```python
from build123d import *

# Parameters (mm, degrees)
SKETCH1_W           = 35.5
SKETCH1_H           = 35
SKETCH1_W_2         = 23.5
SKETCH1_H_2         = 20.5
BOSS_EXTRUDE1_DEPTH = 10
SKETCH1_2_W         = 23.5
SKETCH1_2_H         = 20.5
BOSS_EXTRUDE2_DEPTH = 3.5
SKETCH2_R           = 2.75
SKETCH2_R_2         = 1.5
CUT_EXTRUDE1_DEPTH  = 5.5
SKETCH2_2_R         = 1.5
CUT_EXTRUDE2_DEPTH  = 41.822787754
CUT_EXTRUDE3_START  = -30
SKETCH2_3_R         = 2.75
SKETCH2_3_R_2       = 1.5
CUT_EXTRUDE3_DEPTH  = 5.5
BOSS_EXTRUDE3_DEPTH = 5


with BuildPart() as part:
    # Sketch1 → Boss-Extrude1 (new body)
    with BuildSketch(Plane(origin=(0, 0, 0), x_dir=(1, 0, 0), z_dir=(0, 1, 0))):
        Rectangle(SKETCH1_W, SKETCH1_H)
        Rectangle(SKETCH1_W_2, SKETCH1_H_2, mode=Mode.SUBTRACT)
    extrude(amount=BOSS_EXTRUDE1_DEPTH)

    # Sketch1<2> → Boss-Extrude2 (add)
    with BuildSketch(Plane(origin=(0, 0, 0), x_dir=(1, 0, 0), z_dir=(0, 1, 0))):
        Rectangle(SKETCH1_2_W, SKETCH1_2_H)
    extrude(amount=BOSS_EXTRUDE2_DEPTH)

    # Sketch2 → Cut-Extrude1 (cut)
    # profile 1 of 2: a face of its own
    with BuildSketch(Plane(origin=(17.75, 0, 0), x_dir=(0, 0, -1), z_dir=(1, 0, 0))):
        with Locations((-8, 5.5)):
            Circle(SKETCH2_R)
        with Locations((-8, 5.5)):
            Circle(SKETCH2_R_2, mode=Mode.SUBTRACT)
    # profile 2 of 2: a face of its own
    with BuildSketch(Plane(origin=(17.75, 0, 0), x_dir=(0, 0, -1), z_dir=(1, 0, 0))):
        with Locations((8, 5.5)):
            Circle(SKETCH2_R)
        with Locations((8, 5.5)):
            Circle(SKETCH2_R_2, mode=Mode.SUBTRACT)
    extrude(amount=-CUT_EXTRUDE1_DEPTH, mode=Mode.SUBTRACT)

    # Sketch2<2> → Cut-Extrude2 (cut, through all)
    with BuildSketch(Plane(origin=(17.75, 0, 0), x_dir=(0, 0, -1), z_dir=(1, 0, 0))):
        with Locations((-8, 5.5)):
            Circle(SKETCH2_2_R)
        with Locations((8, 5.5)):
            Circle(SKETCH2_2_R)
    extrude(amount=-CUT_EXTRUDE2_DEPTH, mode=Mode.SUBTRACT)

    # Sketch2<3> → Cut-Extrude3 (cut)
    # profile 1 of 2: a face of its own
    with BuildSketch(Plane(origin=(17.75, 0, 0), x_dir=(0, 0, -1), z_dir=(1, 0, 0)).offset(CUT_EXTRUDE3_START)):
        with Locations((-8, 5.5)):
            Circle(SKETCH2_3_R)
        with Locations((-8, 5.5)):
            Circle(SKETCH2_3_R_2, mode=Mode.SUBTRACT)
    # profile 2 of 2: a face of its own
    with BuildSketch(Plane(origin=(17.75, 0, 0), x_dir=(0, 0, -1), z_dir=(1, 0, 0)).offset(CUT_EXTRUDE3_START)):
        with Locations((8, 5.5)):
            Circle(SKETCH2_3_R)
        with Locations((8, 5.5)):
            Circle(SKETCH2_3_R_2, mode=Mode.SUBTRACT)
    extrude(amount=-CUT_EXTRUDE3_DEPTH, mode=Mode.SUBTRACT)


with BuildPart() as body_2:
    # Mirror1: mirrored copy
    add(part.part.mirror(Plane.ZY.offset(34.75)))


with BuildPart() as part_1:
    add(part.part)

    add(body_2.part)  # Boss-Extrude3 merges body 2
    # Sketch4 → Boss-Extrude3 (add)
    with BuildSketch(Plane(origin=(0, 0, 0), x_dir=(1, 0, 0), z_dir=(0, 1, 0))):
        Polygon((-51.75, -17.5), (-51.75, -67.5), (-17.75, -67.5), (-17.75, -17.5), (17.75, -17.5), (17.75, -97.5), (-87.25, -97.5), (-87.25, -17.5), align=None)
    extrude(amount=BOSS_EXTRUDE3_DEPTH)


solid = part_1.part
```
Work out the finished part from the listing and answer in its coordinate system (mm). A direction names the side the tool comes from. Round coordinates to 2 decimals unless told otherwise and drop trailing zeros. Loops run counter-clockwise (first coordinate to the right, second up) from the corner with the lowest first, then second, coordinate; pieces in that order, holes last. Notation, with made-up numbers: M -23.75,40.25 L -12.75,40.25 A31 cw -12.75,67.25 Z; hole C 73,2 d4. An arc over 180 degrees is marked long. Use CSV: the item, a comma, the result in double quotes.
Q1. Consider L1, parallel to Z at x = -63, y = 6; L2, parallel to X at y = 9, z = -1; L3, parallel to X at y = 3.75, z = 15. Determine where each line is inside the solid, lowest interval first.
Determined:
L1,"-17.5 to -10.25, 10.25 to 17.5"
L2,"-87.25 to -81.25, -57.75 to -51.75, -17.75 to -11.75, 11.75 to 17.75"
L3,"-87.25 to -51.75, -17.75 to 17.75"
Q2. A tool of negligible diameter and unlimited length cuts with its end or side. For faces 4 (the cylindrical face through (-84.54, 4.45, -10.54)), 5 (the cylindrical face through (15.04, 3.06, 6.73)), 6 (the flat face through (-69, 7, -10.25)), 7 (the flat face through (-35, 2, 67.5)), 8 (the flat face through (-57.25, 4, 7)), from which of +Z, -Z, +X, -X, +Y, -Y can it reach the whole face along a straight path? Write none if from no direction.
Determined:
face 4,"-X"
face 5,"+X"
face 6,"+Y"
face 7,"-Z, +Y, -Y"
face 8,"none"
Q3. The mould has two halves that part along Z. Classify faces 1 (the flat face through (-57, 10, 0)), 2 (the flat face through (-69, 7, 17.5)), 3 (the flat face through (-81.75, 4, -9)): pulls with the +Z half, pulls with the -Z half, needs draft (parallel to the pull), parting line crosses it, or undercut.
Determined:
face 1,"needs draft"
face 2,"pulls with the +Z half"
face 3,"undercut"
Q4. Section C-C, the plane z = -8 is taken. State how many separate pieces and enclosed holes the cut face has, then the cut area to 4 significant figures.
Determined:
separate pieces,"6"
enclosed holes,"0"
area,"277.5 mm2"
Q5. Section D-D, the plane x = -49.5 is taken. Determine the outline of the cut face in (y, z).
Determined:
outline,"M 0,67.5 L 5,67.5 L 5,97.5 L 0,97.5 Z"
Q6. Each of these flat-tipped pins is pushed along its axis until it touches: pin 1 (3.5 mm diameter, centred on y = 5.5, z = 8, fed in from +X); pin 2 (3.5 mm diameter, centred on y = 5.5, z = 8, fed in from -X); pin 3 (2.5 mm diameter, centred on x = -42.5, y = 2, fed in from -Z); pin 4 (1.6 mm diameter, centred on y = 5.5, z = -8, fed in from -X). Where does it stop, or does it pass through?
Determined:
pin 1,"x = 12.25"
pin 2,"x = -81.75"
pin 3,"z = 67.5"
pin 4,"through"
Q7. Section A-A, the plane z = 24 is taken. Determine the outline of the cut face in (x, y), then the cut area to 3 significant figures.
Determined:
outline,"M -87.25,0 L -51.75,0 L -51.75,5 L -87.25,5 Z; M -17.75,0 L 17.75,0 L 17.75,5 L -17.75,5 Z"
area,"355 mm2"
Q8. Section B-B, the plane x = 8 is taken. Determine the outline of the cut face in (y, z).
Determined:
outline,"M 0,-17.5 L 10,-17.5 L 10,-10.25 L 3.5,-10.25 L 3.5,10.25 L 10,10.25 L 10,17.5 L 5,17.5 L 5,97.5 L 0,97.5 Z"
